Build history of the part. All positions in model axes, mm. A direction names the side the tool comes from. Round coordinates to 2 decimals unless told otherwise and drop trailing zeros. Order: outer loops, then holes, each group sorted by start corner. A loop starts at its lowest first (then second) coordinate and runs counter-clockwise, first axis right, second up. Notation, with made-up numbers: M 23.25,30 L 36.25,30 A29 cw 36.25,50 Z; hole C 33,-24 d2. An arc over 180 degrees is marked long. One line per question, with ' | ' between items. Start each with the question number.
from build123d import *

# Parameters (mm, degrees)
SKETCH_1_W          = 10
SKETCH_1_H          = 300
SKETCH_2_R          = 1.65
EXTRUDE_1_DEPTH     = 10
SKETCH_3_R          = 10
CUT_EXTRUDE_1_DEPTH = 50


with BuildPart() as part:
    # 草图1 → 旋转1 (revolve)
    with BuildSketch(Plane.XY, mode=Mode.PRIVATE) as revolve_1_sk:
        with Locations((5, 150)):
            Rectangle(SKETCH_1_W, SKETCH_1_H)
    revolve(revolve_1_sk.sketch.rotate(Axis((0, 0, 0), (0, 1, 0)), 90), axis=Axis((0, 0, 0), (0, 1, 0)))

    # 草图2 → 凸台-拉伸1 (add)
    with BuildSketch(Plane(origin=(0, 300, 0), x_dir=(1, 0, 0), z_dir=(0, 1, 0))):
        with Locations(Location((7, 0, 0), (0, 0, 90))):
            Circle(SKETCH_2_R)
        with Locations(Location((0, -7, 0), (0, 0, 90))):
            Circle(SKETCH_2_R)
        with Locations(Location((-7, 0, 0), (0, 0, 90))):
            Circle(SKETCH_2_R)
        with Locations(Location((0, 7, 0), (0, 0, 90))):
            Circle(SKETCH_2_R)
    extrude(amount=EXTRUDE_1_DEPTH)

    # 草图3 → 切除-拉伸1 (cut)
    with BuildSketch(Plane.XZ):
        with Locations(Location((0, 0, 0), (0, 0, 270))):
            Circle(SKETCH_3_R)
    extrude(amount=-CUT_EXTRUDE_1_DEPTH, mode=Mode.SUBTRACT)


solid = part.part
Item 1: Cut at A-A on y = 166. Write the cut outline in (x, z), then the cut area to 3 significant figures.
Item 2: Wall check: line 1 along Y through (x, z) = (3.25, 9.25); line 2 along X through (y, z) = (205.5, 1); line 3 along Z through (x, y) = (0.25, 260.5). Give the ranges that are in metal, low to high. Write a range as [from, to].
Item 3: Flat gauge pins, fed straight in: pin 1 (1.5 mm diameter, centred on y = 122.5, z = 4.5, fed in from -X); pin 2 (2 mm diameter, centred on x = -6.5, y = 227.5, fed in from +Z); pin 3 (2 mm diameter, centred on x = -3, z = 8, fed in from +Y). Where does each tip first touch, or does it go through?
Item 4: Tool access for faces 1 (the face through (0, 300, 0)), 2 (the face through (0, 177, 10)): list every direction of +Z, -Z, +X, -X, +Y, -Y with a clear straight run to the whole face (end or side of a thin tool).
Results found:
1) outline: C 0,0 d20 | area: 314 mm^2
2) line 1: y = [50, 300] | line 2: x = [-9.95, 9.95] | line 3: z = [-10, 10]
3) pin 1: stops at x = -9.27 | pin 2: stops at z = 8.35 | pin 3: stops at y = 300
4) face 1: +Y | face 2: +Y, -Y
